Autodesk Inventor part; units mm, degrees
ref_plane "YZ Plane" through (0, 0, 0) normal (1, 0, 0) x (0, 1, 0)
ref_plane "XZ Plane" through (0, 0, 0) normal (0, 1, 0) x (-1, 0, 0)
ref_plane "XY Plane" through (0, 0, 0) normal (0, 0, 1) x (1, 0, 0)
sketch "Sketch1" plane through (0, 0, 0) normal (0, 1, 0) x (-1, 0, 0)
  line L0 (-10, -15) -> (10, -15)
  line L1 (10, -15) -> (10, 15)
  line L2 (10, 15) -> (-10, 15)
  line L3 (-10, 15) -> (-10, -15)
  line L4 (-10, -15) -> (10, 15) construction
  line L5 (10, -15) -> (-10, 15) construction
  point P0 (0, 0)
  dimension "d0" = 20
  dimension "d1" = 30
extrude "Extrusion1" add sketch "Sketch1" along normal blind 5
sketch "Sketch2" plane through (0, 5, 0) normal (0, 1, 0) x (1, 0, 0)
  line L0 (-10, -15) -> (10, -15)
  line L1 (0, -15) -> (0, 15)
  line L2 (10, 15) -> (-10, 15)
  point P0 (0, 0)
  point P1 (0, -19.7357)
  point P2 (0, -11.8278)
  point P3 (0, -3.988)
  point P4 (0, 4.0562)
  point P5 (0, 11.7596)
  point P6 (0, 20.6901)
hole "Hole1" at (0, 5, 19.7357) at (0, 5, 0) direction (0, -1, 0) diameter 3.4 end through all counterbore diameter 6.5 counterbore depth 3.4
sketch "Sketch3" plane through (0, 5, 0) normal (0, 1, 0) x (1, 0, 0)
  point P0 (0, 0)
  point P1 (-0.6602, -10.4342)
hole "Hole2" at (-0.6602, 5, 10.4342) direction (0, -1, 0) diameter 2.459 end through all
properties part number "Tap_Test"
The listing builds one solid part. Answer for the finished solid, in the listing's coordinates (mm). A direction names the side the tool comes from. Coordinates: 2 decimals unless noted, no trailing zeros. Write each loop counter-clockwise with the first axis right and the second up, starting at its lowest first coordinate (ties: lowest second). Pieces come first, ordered by that corner, then holes. Notation, with made-up numbers: M 57.5,48 L 79.5,48 A21 ccw 79.5,70 Z; hole C 88,-21.5 d2. An arc over 180 degrees is marked long. Use a Markdown table: item, result. Add a question column.
1. Section A-A (z = 0) is taken. Give the vertices of the cut face in (x, y).
2. For a pull along X with two mould halves and no side action, classify faces 3 (the flat face through (0, 5, 4)), 4 (the cylindrical face through (1.978, 3.276, -2.579)), 5 (the flat face through (-10, 2, 0)) as +X half, -X half, draft (parallel to the pull), parting line (faces both ways), or undercut.
3. Given P1, Ø3, axis at x = -0.5, z = 0.5, coming from the +Y side; P2, Ø3, axis at x = 0, z = 0, coming from the +Y side, each flat-ended and moving along its own axis, determine where each tip first touches the part or whether it passes through.
4. Section D-D (z = 11.25) is taken. Give the vertices of the cut face in (x, y), plus the area to 3 significant figures.
5. Straight lines are drawn through the part: line 1 along X through (y, z) = (3.95, 0); line 2 along Z through (x, y) = (0, 3.4); line 3 along Z through (x, y) = (0, 0.3). For each, find the intervals that lie inside material, in ascending order. Write a range as [from, to].
6. Which of the six approach directions +Z, -Z, +X, -X, +Y, -Y give full straight-line access (tool end or side, diameter ignored) to faces 1 (the flat face through (1.4, 1.6, 1.4)), 2 (the cylindrical face through (1.66, 0.79, -0.37))?
7. Section B-B (x = 0) is taken. Give the vertices of the cut face in (y, z).
8. Section C-C (y = 3) is taken. Give the vertices of the cut face in (x, z).
Data:
| question | item | result |
|---|---|---|
| 1 | outline | M -10,0 L -1.7,0 L -1.7,1.6 L -3.25,1.6 L -3.25,5 L -10,5 Z; M 1.7,0 L 10,0 L 10,5 L 3.25,5 L 3.25,1.6 L 1.7,1.6 Z |
| 2 | face 3 | draft |
| 2 | face 4 | undercut |
| 2 | face 5 | -X half |
| 3 | P1 | stops at y = 1.6 |
| 3 | P2 | passes through |
| 4 | outline | M -10,0 L -1.58,0 L -1.58,5 L -10,5 Z; M 0.26,0 L 10,0 L 10,5 L 0.26,5 Z |
| 4 | area | 90.8 mm2 |
| 5 | line 1 | x = [-10, -3.25], [3.25, 10] |
| 5 | line 2 | z = [-15, -3.25], [3.25, 9.4], [11.47, 15] |
| 5 | line 3 | z = [-15, -1.7], [1.7, 9.4], [11.47, 15] |
| 6 | face 1 | +Y |
| 6 | face 2 | +Y, -Y |
| 7 | outline | M 0,-15 L 5,-15 L 5,-3.25 L 1.6,-3.25 L 1.6,-1.7 L 0,-1.7 Z; M 0,1.7 L 1.6,1.7 L 1.6,3.25 L 5,3.25 L 5,9.4 L 0,9.4 Z; M 0,11.47 L 5,11.47 L 5,15 L 0,15 Z |
| 8 | outline | M -10,-15 L 10,-15 L 10,15 L -10,15 Z; hole C 0,0 d6.5; hole C -0.66,10.43 d2.46 |
